Geometry check sheet. Reference: the model listing, model coordinates, mm. A direction names the side the tool comes from. Coordinates: 2 decimals unless noted, no trailing zeros. Order: outer loops, then holes, each group sorted by start corner. A loop starts at its lowest first (then second) coordinate and runs counter-clockwise, first axis right, second up. Notation, with made-up numbers: (85.25, -37) - (95.25, -37) arc R23 cw to (95.25, -1) - close; hole circle Ø11 at (83, 83). An arc over 180 degrees is marked (long way). Use CSV: the item, a comma, the result in double quotes. Start each with the question number.
1) Tool access check on faces 3 (the flat face through (0, 2.5, 2)), 4 (the cylindrical face through (-1.57, 0.45, 6.96)). Record the directions out of +Z, -Z, +X, -X, +Y, -Y that give a thin tool (end or side, any length) a straight path to the whole face; none if there is none.
2) Thickness scan on probe 1 along X at (y, z) = (-0.05, 8.5); probe 2 along Z at (x, y) = (-5.25, -0.75); probe 3 along X at (y, z) = (0.5, 6.5). Record the ranges inside material, lowest first. Write a range as [from, to].
3) Sectioned sample at D-D, the plane x = 0.5. Record the cut outline in (y, z).
4) Sectioned sample at C-C, the plane z = 3. Record the cut outline in (x, y).
5) Sectioned sample at A-A, the plane z = 7. Record the cut outline in (x, y), and give its area (3 significant figures).
6) Draft check along X on faces 1 (the cylindrical face through (5.386, -0.575, 6.958)), 2 (the cylindrical face through (0.056, -2.215, 0.301)). Enter one of: released by +X, released by -X, zero draft, split by the parting line, or undercut.
7) Depth check by flat-ended pin: P1, Ø2, axis at x = 3.5, z = 7, coming from the -Y side; P2, Ø1.5, axis at x = 1.5, y = -1, coming from the +Z side. Enter the tip coordinate at first touch or a pass-through.
8) Sectioned sample at B-B, the plane x = -3. Record the cut outline in (y, z).
from build123d import *

# Parameters (mm, degrees)
F0_R     = 1.5
F1_DEPTH = 10
F2_DEPTH = 4
F3_R     = 1


with BuildPart() as f1:
    # F0 (on Top) → F1 (new body)
    with BuildSketch(Plane.XY):
        with Locations((4, 0)):
            Circle(F0_R)
    extrude(amount=F1_DEPTH)



with BuildPart() as f1b:
    # F0 (on Top) → F1, piece 2 (new body)
    with BuildSketch(Plane.XY):
        with Locations((-3, 0)):
            Circle(F0_R)
    extrude(amount=F1_DEPTH)


with BuildPart() as f1_1:
    add(f1.part)

    add(f1b.part)  # F2 merges F1b
    # F0 (on Top) → F2 (join)
    with BuildSketch(Plane.XY):
        with BuildLine():
            Line((4, 2.5), (-4, 2.5))
            ThreePointArc((-4, 2.5), (-5.767766953, 1.767766953), (-6.5, 0))
            ThreePointArc((-6.5, 0), (-5.767766953, -1.767766953), (-4, -2.5))
            Line((-4, -2.5), (4, -2.5))
            ThreePointArc((4, -2.5), (5.767766953, -1.767766953), (6.5, 0))
            ThreePointArc((6.5, 0), (5.767766953, 1.767766953), (4, 2.5))
        make_face()
        with Locations((-3, 0)):
            Circle(F0_R, mode=Mode.SUBTRACT)
        with Locations((4, 0)):
            Circle(F0_R, mode=Mode.SUBTRACT)
    extrude(amount=F2_DEPTH)

    # F3
    f3_edges = [f1_1.edges().sort_by_distance(p)[0] for p in [
        (0, 2.5, 0),
        (-6.5, 0, 0),
    ]]
    fillet(f3_edges, radius=F3_R)


solid = f1_1.part
Evaluation:
1,face 3,"+Z, -Z, +X, -X, +Y"
1,face 4,"+Z"
2,probe 1,"[-4.5, -1.5], [2.5, 5.5]"
2,probe 2,"[0, 4]"
2,probe 3,"[-4.41, -1.59], [2.59, 5.41]"
3,outline,"(-2.5, 1) arc R1 ccw to (-1.5, 0) - (1.5, 0) arc R1 ccw to (2.5, 1) - (2.5, 4) - (-2.5, 4) - close"
4,outline,"(-4, -2.5) - (4, -2.5) arc R2.5 ccw to (4, 2.5) - (-4, 2.5) arc R2.5 ccw to start"
5,outline,"circle Ø3 at (-3, 0); circle Ø3 at (4, 0)"
5,area,"14.1 mm²"
6,face 1,"undercut"
6,face 2,"zero draft"
7,P1,"y = -1.5"
7,P2,"z = 4"
8,outline,"(-2.5, 1) arc R1 ccw to (-1.5, 0) - (1.5, 0) arc R1 ccw to (2.5, 1) - (2.5, 4) - (1.5, 4) - (1.5, 10) - (-1.5, 10) - (-1.5, 4) - (-2.5, 4) - close"
